```python
from build123d import *

# Parameters (mm, degrees)
SKETCH1_W           = 91.44
SKETCH1_H           = 91.44
BOSS_EXTRUDE1_DEPTH = 3.175
SKETCH2_W           = 80.01
SKETCH2_H           = 80.01
BOSS_EXTRUDE2_DEPTH = 3.048
CUT_EXTRUDE1_DEPTH  = 65.956620363
SKETCH4_R           = 2.159
CUT_EXTRUDE2_DEPTH  = 65.956620363
FILLET1_R           = 2.54
SKETCH5_R           = 1.5875
CUT_EXTRUDE3_DEPTH  = 65.956620363


with BuildPart() as part:
    # Sketch1 → Boss-Extrude1 (new body)
    with BuildSketch(Plane(origin=(0, 0, 0), x_dir=(1, 0, 0), z_dir=(0, 1, 0))):
        Rectangle(SKETCH1_W, SKETCH1_H)
    extrude(amount=BOSS_EXTRUDE1_DEPTH)

    # Sketch2 → Boss-Extrude2 (add)
    with BuildSketch(Plane.XZ):
        Rectangle(SKETCH2_W, SKETCH2_H)
    extrude(amount=BOSS_EXTRUDE2_DEPTH)

    # Sketch3 → Cut-Extrude1 (cut, through all)
    with BuildSketch(Plane.XZ.offset(3.048)):
        Polygon((-24.13, 40.005), (-40.005, 24.13), (-40.005, -24.13), (-24.13, -40.005), (24.13, -40.005), (40.005, -24.13), (40.005, 24.13), (24.13, 40.005), align=None)
    extrude(amount=-CUT_EXTRUDE1_DEPTH, mode=Mode.SUBTRACT)

    # Sketch4 → Cut-Extrude2 (cut, through all)
    with BuildSketch(Plane.XZ.offset(3.048)):
        with Locations(Location((-36.068, 36.068, 0), (0, 0, 270))):
            Circle(SKETCH4_R)
        with Locations(Location((36.068, 36.068, 0), (0, 0, 270))):
            Circle(SKETCH4_R)
        with Locations(Location((36.068, -36.068, 0), (0, 0, 270))):
            Circle(SKETCH4_R)
        with Locations(Location((-36.068, -36.068, 0), (0, 0, 270))):
            Circle(SKETCH4_R)
    extrude(amount=-CUT_EXTRUDE2_DEPTH, mode=Mode.SUBTRACT)

    # Fillet1
    fillet1_edges = [part.edges().sort_by_distance(p)[0] for p in [
        (40.005, -1.524, -40.005),
        (40.005, -1.524, 40.005),
        (-40.005, -1.524, 40.005),
        (-40.005, -1.524, -40.005),
    ]]
    fillet(fillet1_edges, radius=FILLET1_R)

    # Sketch5 → Cut-Extrude3 (cut, through all)
    with BuildSketch(Plane(origin=(0, 3.175, 0), x_dir=(1, 0, 0), z_dir=(0, 1, 0))):
        with Locations(Location((-42.545, 42.545, 0), (0, 0, 270))):
            Circle(SKETCH5_R)
        with Locations(Location((42.545, 42.545, 0), (0, 0, 270))):
            Circle(SKETCH5_R)
        with Locations(Location((42.545, -42.545, 0), (0, 0, 270))):
            Circle(SKETCH5_R)
        with Locations(Location((-42.545, -42.545, 0), (0, 0, 270))):
            Circle(SKETCH5_R)
    extrude(amount=-CUT_EXTRUDE3_DEPTH, mode=Mode.SUBTRACT)


solid = part.part
```
The listing builds one solid part. Answer for the finished solid, in the listing's coordinates (mm). A direction names the side the tool comes from. Give positions to 0.01 mm unless a question says otherwise; leave off trailing zeros. Order: outer loops, then holes, each group sorted by start corner. A loop starts at its lowest first (then second) coordinate and runs counter-clockwise, first axis right, second up. Notation, with made-up numbers: (17, 46.25) -> (75, 46.25) arc R26 cw to (75, 69.25) -> close; hole circle Ø10 at (56, 56.5). An arc over 180 degrees is marked (long way). Answer as a JSON object with one key per item and string values. Group by question number.
Item 1: Determine the mould class of faces 1 (the flat face through (-40.005, -2, -31)), 2 (the cylindrical face through (37.888, 0.02, -37.229)), 3 (the cylindrical face through (-41.2, 1.6, -41.7)), 4 (the flat face through (-31, -2, 40.005)) for opening direction Z: pulls with the +Z half, pulls with the -Z half, needs draft (parallel to the pull), parting line crosses it, or undercut.
Item 2: A tool of negligible diameter and unlimited length cuts with its end or side. For faces 5 (the cylindrical face through (-39.28, -1.55, -39.24)), 6 (the flat face through (0, 2, -40.005)), 7 (the flat face through (40.005, -2, 31)), 8 (the cylindrical face through (-39.28, -1.55, 39.24)), from which of +Z, -Z, +X, -X, +Y, -Y can it reach the whole face along a straight path? Write none if from no direction.
Item 3: The part is cut by section A-A on z = 5. Write down the section's boundary in (x, y) (3 decimals), and give its area (3 significant figures).
Item 4: The part is cut by section B-B on y = -2. Write down the section's boundary in (x, z) (3 decimals), and give its area (3 significant figures).
Item 5: The part is cut by section C-C on x = -15. Write down the section's boundary in (y, z) (3 decimals), and give its area (3 significant figures).
Item 6: Consider L1, parallel to X at y = 0.75, z = 42.5; L2, parallel to Z at x = -19, y = 2.25 (3 decimals); L3, parallel to X at y = 2.25, z = -35 (3 decimals). Determine where each line is inside the solid, lowest interval first. Write a range as from..to.
Item 7: Flat-ended cylindrical pins translate along their axes: pin 1 (2.5 mm diameter, centred on x = -42.545, z = -42.545, fed in from +Y); pin 2 (1.5 mm diameter, centred on y = -2, z = 30.5, fed in from -X) (3 decimals); pin 3 (0.9 mm diameter, centred on x = -29.5, y = -1.5, fed in from +Z) (3 decimals); pin 4 (0.9 mm diameter, centred on x = 31, y = -2, fed in from -Z) (3 decimals). Find the tip coordinate at first contact, or state that the pin passes through.
Result set:
{
 "1": {"face 1": "needs draft", "face 2": "undercut", "face 3": "undercut", "face 4": "pulls with the +Z half"},
 "2": {"face 5": "-Z, -X, -Y", "face 6": "+Y, -Y", "face 7": "+Z, -Z, +X, -Y", "face 8": "+Z, -X, -Y"},
 "3": {"outline": "(-45.72, 0) -> (-40.005, 0) -> (-40.005, 3.175) -> (-45.72, 3.175) -> close; (40.005, 0) -> (45.72, 0) -> (45.72, 3.175) -> (40.005, 3.175) -> close", "area": "36.3 mm²"},
 "4": {"outline": "(-40.005, -37.465) arc R2.54 ccw to (-37.465, -40.005) -> (-24.13, -40.005) -> (-40.005, -24.13) -> close; (-40.005, 24.13) -> (-24.13, 40.005) -> (-37.465, 40.005) arc R2.54 ccw to (-40.005, 37.465) -> close; (24.13, -40.005) -> (37.465, -40.005) arc R2.54 ccw to (40.005, -37.465) -> (40.005, -24.13) -> close; (24.13, 40.005) -> (40.005, 24.13) -> (40.005, 37.465) arc R2.54 ccw to (37.465, 40.005) -> close; hole circle Ø4.318 at (-36.068, -36.068); hole circle Ø4.318 at (-36.068, 36.068); hole circle Ø4.318 at (36.068, -36.068); hole circle Ø4.318 at (36.068, 36.068)", "area": "440 mm²"},
 "5": {"outline": "(0, -45.72) -> (3.175, -45.72) -> (3.175, -40.005) -> (0, -40.005) -> close; (0, 40.005) -> (3.175, 40.005) -> (3.175, 45.72) -> (0, 45.72) -> close", "area": "36.3 mm²"},
 "6": {"L1": "-45.72..-44.13, -40.96..40.96, 44.13..45.72", "L2": "-45.72..-40.005, 40.005..45.72", "L3": "-45.72..-37.944, -34.192..-29.135, 29.135..34.192, 37.944..45.72"},
 "7": {"pin 1": "through", "pin 2": "x = -40.005", "pin 3": "z = 40.005", "pin 4": "z = -40.005"}
}
